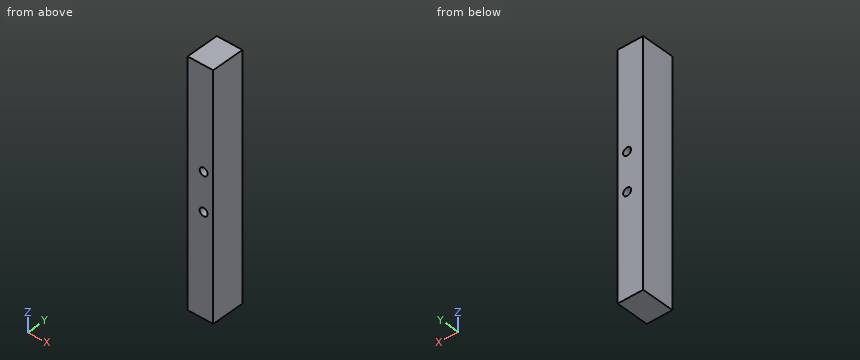
Autodesk Inventor part; units mm, degrees
ref_plane "YZ Plane" through (0, 0, 0) normal (1, 0, 0) x (0, 1, 0)
ref_plane "XZ Plane" through (0, 0, 0) normal (0, 1, 0) x (-1, 0, 0)
ref_plane "XY Plane" through (0, 0, 0) normal (0, 0, 1) x (1, 0, 0)
sketch "Sketch1" plane through (0, 0, 0) normal (0, 0, 1) x (1, 0, 0)
  line L0 (-8.5, 0) -> (8.5, 0)
  line L1 (8.5, 0) -> (8.5, 22)
  line L2 (8.5, 22) -> (-8.5, 22)
  line L3 (-8.5, 22) -> (-8.5, 0)
  point P0 (0, 0)
  point P1 (0, 0)
  dimension "d0" = 22
  dimension "d1" = 17
extrude "Extrusion1" add sketch "Sketch1" along normal mid plane 160
sketch "Sketch2" plane through (-8.5, 22, -80) normal (0, 1, 0) x (1, 0, 0)
  line L0 (17, 0) -> (17, -160)
  line L1 (10.65, -92.7) -> (10.65, -80)
  point P0 (17, -80)
  dimension "d4" = 6.35
  dimension "d16" = 12.7
hole "Hole1" at (2.15, 22, 12.7) direction (0, -1, 0) diameter 5.2578 end through all
pattern_linear "Rectangular Pattern1" count 2 spacing 25.4 along (0, 0, -1) of "Hole1"
properties part number "PWTR-0041" material "Stainless Steel, 303"
Source: CAD feature listing. Evaluate the final solid. Frame: model axes, mm. Give positions to 0.01 mm unless a question says otherwise; leave off trailing zeros. Write each loop counter-clockwise with the first axis right and the second up, starting at its lowest first coordinate (ties: lowest second). Pieces come first, ordered by that corner, then holes.
1. Section query B-B (z = -12.7). Return the cut outline in (x, y), then the cut area to 3 significant figures.
2. Section query D-D (z = 13). Return the cut outline in (x, y), then the cut area to 3 significant figures.
3. Material intervals for line 1 along Z through (x, y) = (2.15, 11.25); line 2 along X through (y, z) = (15, -12.7); line 3 along Z through (x, y) = (1.5, 21.25), sorted ascending.
4. Section query A-A (x = 2.15). Return the cut outline in (y, z), then the cut area to 3 significant figures.
5. Section query C-C (y = 14). Return the cut outline in (x, z).
Output values:
1. outline: (-8.5, 0) - (-0.48, 0) - (-0.48, 22) - (-8.5, 22) - close; (4.78, 0) - (8.5, 0) - (8.5, 22) - (4.78, 22) - close
1. area: 258 mm2
2. outline: (-8.5, 0) - (-0.46, 0) - (-0.46, 22) - (-8.5, 22) - close; (4.76, 0) - (8.5, 0) - (8.5, 22) - (4.76, 22) - close
2. area: 259 mm2
3. line 1: z = -80 to -15.33, -10.07 to 10.07, 15.33 to 80
3. line 2: x = -8.5 to -0.48, 4.78 to 8.5
3. line 3: z = -80 to -15.25, -10.15 to 10.15, 15.25 to 80
4. outline: (0, -80) - (22, -80) - (22, -15.33) - (0, -15.33) - close; (0, -10.07) - (22, -10.07) - (22, 10.07) - (0, 10.07) - close; (0, 15.33) - (22, 15.33) - (22, 80) - (0, 80) - close
4. area: 3,290 mm2
5. outline: (-8.5, -80) - (8.5, -80) - (8.5, 80) - (-8.5, 80) - close; hole circle Ø5.26 at (2.15, -12.7); hole circle Ø5.26 at (2.15, 12.7)
